Geometry: final body of the model. Coordinates: model frame, mm. A direction names the side the tool comes from. Give positions to 0.01 mm unless a question says otherwise; leave off trailing zeros. Write each loop counter-clockwise with the first axis right and the second up, starting at its lowest first coordinate (ties: lowest second). Pieces come first, ordered by that corner, then holes.
from build123d import *

# Parameters (mm, degrees)
EXTRUDE_1_DEPTH     = 14
CUT_EXTRUDE_1_DEPTH = 44
SKETCH_3_W          = 6.2
SKETCH_3_H          = 6.2
CUT_EXTRUDE_2_DEPTH = 4
SKETCH_4_R          = 4
CUT_EXTRUDE_3_DEPTH = 5
SKETCH_5_R          = 2.6
CUT_EXTRUDE_4_DEPTH = 5


with BuildPart() as part:
    # 草图1 → 凸台-拉伸1 (new body)
    with BuildSketch(Plane.XY):
        Polygon((-15, 22), (-15, -22), (15, -22), (15, 22), (0, 22), align=None)
    extrude(amount=EXTRUDE_1_DEPTH)

    # 草图2 → 切除-拉伸1 (cut)
    with BuildSketch(Plane(origin=(0, 22, 0), x_dir=(1, 0, 0), z_dir=(0, 1, 0))):
        Polygon((-15, 0), (-15, -14), (-10, -4), (-3.1, -4), (-3.1, 0), align=None)
        Polygon((3.1, -4), (10, -4), (15, -14), (15, 0), (3.1, 0), align=None)
    extrude(amount=-CUT_EXTRUDE_1_DEPTH, mode=Mode.SUBTRACT)

    # 草图3 → 切除-拉伸2 (cut)
    with BuildSketch(Plane(origin=(0, 0, 0), x_dir=(-1, 0, 0), z_dir=(0, 0, -1))):
        Rectangle(SKETCH_3_W, SKETCH_3_H)
    extrude(amount=-CUT_EXTRUDE_2_DEPTH, mode=Mode.SUBTRACT)

    # 草图4 → 切除-拉伸3 (cut)
    with BuildSketch(Plane.XY.offset(14)):
        Circle(SKETCH_4_R)
    extrude(amount=-CUT_EXTRUDE_3_DEPTH, mode=Mode.SUBTRACT)

    # 草图5 → 切除-拉伸4 (cut)
    with BuildSketch(Plane.XY.offset(9)):
        Circle(SKETCH_5_R)
    extrude(amount=-CUT_EXTRUDE_4_DEPTH, mode=Mode.SUBTRACT)


solid = part.part
Q1. Pull-direction query (X, two-part tool) for faces 6 (the flat face through (0, 5, 14)), 7 (the flat face through (-3.1, -12, 2)), 8 (the cylindrical face through (-0.867, -3.905, 11.535)); classes: released by +X, released by -X, zero draft, split by the parting line, or undercut.
Filled sheet:
face 6: zero draft
face 7: released by -X
face 8: undercut
Q2. Pin query (flat end, axial travel): P1, Ø8, axis at y = -13, z = 7.5, coming from the +X side; P2, Ø3, axis at y = -3.5, z = 12, coming from the -X side; P3, Ø1.2, axis at y = 16, z = 2, coming from the +X side. Return the tip coordinate at first contact, or that it passes through.
Filled sheet:
P1: stops at x = 13.75
P2: stops at x = -14.75
P3: stops at x = 3.1
Q3. Ray query, line 1 along Y through (x, z) = (0, 6.8); line 2 along Y through (x, z) = (0, 10.55); line 3 along Z through (x, y) = (8.75, -10). Return the intervals inside material, ascending.
Filled sheet:
line 1: y = -22 to -2.6, 2.6 to 22
line 2: y = -22 to -4, 4 to 22
line 3: z = 4 to 14
Q4. Access query for faces 1 (the flat face through (0, 13, 0)), 2 (the flat face through (3.1, -12, 2)), 3 (the flat face through (-3.1, 13, 2)), 4 (the flat face through (3, 0, 9)), 5 (the flat face through (0, -3.1, 2)). Directions: +Z, -Z, +X, -X, +Y, -Y. A direction counts if a zero-diameter tool reaches every point of the face in a straight line with its end or side. Return the directions, or none.
Filled sheet:
face 1: -Z, +X, -X, +Y, -Y
face 2: -Z, +X, +Y, -Y
face 3: -Z, -X, +Y, -Y
face 4: +Z
face 5: -Z, +X, -X
Q5. Section A-A on x = 0. Output: boundary loops of the cut face in (y, z), plus the area to 3 significant figures.
Filled sheet:
outline: (-22, 0) - (-3.1, 0) - (-3.1, 4) - (-2.6, 4) - (-2.6, 9) - (-4, 9) - (-4, 14) - (-22, 14) - close; (2.6, 4) - (3.1, 4) - (3.1, 0) - (22, 0) - (22, 14) - (4, 14) - (4, 9) - (2.6, 9) - close
area: 525 mm2
Q6. Section D-D on z = 6. Output: boundary loops of the cut face in (x, y), plus the area to 3 significant figures.
Filled sheet:
outline: (-11, -22) - (11, -22) - (11, 22) - (-11, 22) - close; hole circle Ø5.2 at (0, 0)
area: 947 mm2
Q7. Section B-B on y = 0. Output: boundary loops of the cut face in (x, z).
Filled sheet:
outline: (-15, 14) - (-10, 4) - (-2.6, 4) - (-2.6, 9) - (-4, 9) - (-4, 14) - close; (2.6, 4) - (10, 4) - (15, 14) - (4, 14) - (4, 9) - (2.6, 9) - close
Q8. Section C-C on z = 3.25. Output: boundary loops of the cut face in (x, y).
Filled sheet:
outline: (-3.1, -22) - (3.1, -22) - (3.1, -3.1) - (-3.1, -3.1) - close; (-3.1, 3.1) - (3.1, 3.1) - (3.1, 22) - (-3.1, 22) - close
